Here's the drawing with two shaded views (mm, measured from the low corner). I have some questions. Coordinates: 2 decimals unless noted, no trailing zeros. Loops run counter-clockwise (first coordinate to the right, second up) from the corner with the lowest first, then second, coordinate; pieces in that order, holes last. Notation, with made-up numbers: (-21.5, 61.25) - (29.5, 61.25) arc R34 cw to (29.5, 95.25) - close; hole circle Ø5 at (57, 12.5). An arc over 180 degrees is marked (long way). One line per item, written item: value. Start each with the question number.
(1) If we section it at C-C on y = 8.25: Write out the boundary of the cut face in (x, z).
(2) I'm going to push flat-ended pins straight in: P1, Ø2, axis at x = 4.5, y = 1, coming from the +Z side; P2, Ø12, axis at x = 17.5, z = 17.5, coming from the -Y side; P3, Ø2, axis at y = 8.5, z = 8, coming from the +X side; P4, Ø1, axis at y = 2, z = 11, coming from the +X side. Where does each tip first touch, or does it pass through?
(3) If we mould it in two halves opening along X, with no side actions, what happens to the marked faces 1, 2 and 3? For each: pulls with the +X half, pulls with the -X half, needs draft (parallel to the pull), parting line crosses it, or undercut.
(4) If we section it at A-A on x = 17.5: Write out the boundary of the cut face in (y, z).
(5) If we section it at D-D on x = 4: Write out the boundary of the cut face in (y, z), then the cut area to 3 significant figures.
(6) If I drill on line 1 along Y through (x, z) = (9, 3); line 2 along X through (y, z) = (5.5, 17.5); line 3 along X through (y, z) = (7.75, 17.5), over which ranges is the centre line in solid material (lowest first)? Write a range as from..to.
(7) If we section it at B-B on z = 23: Write out the boundary of the cut face in (x, y), then the cut area to 3 significant figures.
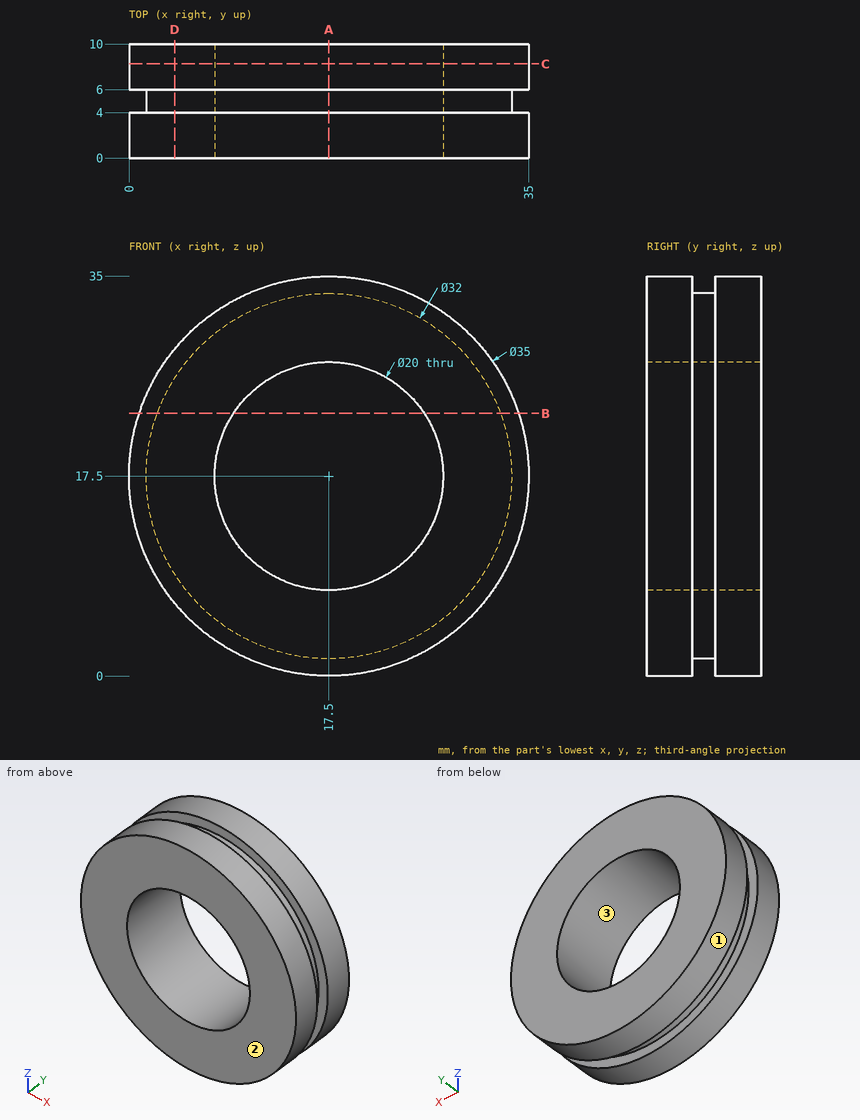
Values:
1. outline: circle Ø35 at (17.5, 17.5); hole circle Ø20 at (17.5, 17.5)
2. P1: stops at z = 30.24
2. P2: passes through
2. P3: stops at x = 32.8
2. P4: stops at x = 33.94
3. face 1: parting line crosses it
3. face 2: needs draft
3. face 3: undercut
4. outline: (0, 0) - (4, 0) - (4, 1.5) - (6, 1.5) - (6, 0) - (10, 0) - (10, 7.5) - (0, 7.5) - close; (0, 27.5) - (10, 27.5) - (10, 35) - (6, 35) - (6, 33.5) - (4, 33.5) - (4, 35) - (0, 35) - close
5. outline: (0, 6.36) - (4, 6.36) - (4, 8.91) - (6, 8.91) - (6, 6.36) - (10, 6.36) - (10, 28.64) - (6, 28.64) - (6, 26.09) - (4, 26.09) - (4, 28.64) - (0, 28.64) - close
5. area: 213 mm2
6. line 1: y = 0..4, 6..10
6. line 2: x = 1.5..7.5, 27.5..33.5
6. line 3: x = 0..7.5, 27.5..35
7. outline: (0.89, 0) - (9.15, 0) - (9.15, 10) - (0.89, 10) - (0.89, 6) - (2.48, 6) - (2.48, 4) - (0.89, 4) - close; (25.85, 0) - (34.11, 0) - (34.11, 4) - (32.52, 4) - (32.52, 6) - (34.11, 6) - (34.11, 10) - (25.85, 10) - close
7. area: 159 mm2
